```python
from build123d import *

# Parameters (mm, degrees)
SKETCH1_R           = 9
BOSS_EXTRUDE1_DEPTH = 14
SKETCH2_R           = 27.5
SKETCH2_R_2         = 15
BOSS_EXTRUDE2_DEPTH = 22.5
SKETCH3_R           = 27.5
SKETCH3_R_2         = 15
BOSS_EXTRUDE3_DEPTH = 22.5
BOSS_EXTRUDE4_DEPTH = 7.5
BOSS_EXTRUDE9_DEPTH = 7.5


with BuildPart() as part:
    # Sketch1 → Boss-Extrude1 (new body)
    with BuildSketch(Plane(origin=(0, 0, 0), x_dir=(1, 0, 0), z_dir=(0, 1, 0))):
        with BuildLine():
            Line((153.801246265, 0), (225.801246265, 0))
            ThreePointArc((225.801246265, 0), (232.872314076, 2.928932188), (235.801246265, 10))
            Line((235.801246265, 10), (235.801246265, 132))
            ThreePointArc((235.801246265, 132), (232.872314076, 139.071067812), (225.801246265, 142))
            Line((225.801246265, 142), (153.801246265, 142))
            ThreePointArc((153.801246265, 142), (146.730178453, 139.071067812), (143.801246265, 132))
            Line((143.801246265, 132), (143.801246265, 10))
            ThreePointArc((143.801246265, 10), (146.730178453, 2.928932188), (153.801246265, 0))
        make_face()
        with Locations(Location((164.801246265, 22.845020392, 0), (0, 0, 270))):
            Circle(SKETCH1_R, mode=Mode.SUBTRACT)
        with Locations(Location((214.801246265, 22.845020392, 0), (0, 0, 270))):
            Circle(SKETCH1_R, mode=Mode.SUBTRACT)
        with Locations(Location((214.801246265, 118.829727622, 0), (0, 0, 270))):
            Circle(SKETCH1_R, mode=Mode.SUBTRACT)
        with Locations(Location((164.801246265, 118.829727622, 0), (0, 0, 270))):
            Circle(SKETCH1_R, mode=Mode.SUBTRACT)
    extrude(amount=-BOSS_EXTRUDE1_DEPTH)



with BuildPart() as body_2:
    # Sketch2 → Boss-Extrude2 (new body)
    with BuildSketch(Plane.XY.offset(-71)):
        with Locations(Location((189.801246265, 58, 0), (0, 0, 180))):
            Circle(SKETCH2_R)
        with Locations(Location((189.801246265, 58, 0), (0, 0, 180))):
            Circle(SKETCH2_R_2, mode=Mode.SUBTRACT)
    extrude(amount=BOSS_EXTRUDE2_DEPTH)

    # Sketch3 → Boss-Extrude3 (add)
    with BuildSketch(Plane(origin=(0, 0, -71), x_dir=(-1, 0, 0), z_dir=(0, 0, -1))):
        with Locations((-189.801246265, 58)):
            Circle(SKETCH3_R)
        with Locations((-189.801246265, 58)):
            Circle(SKETCH3_R_2, mode=Mode.SUBTRACT)
    extrude(amount=BOSS_EXTRUDE3_DEPTH)


with BuildPart() as part_1:
    add(part.part)

    add(body_2.part)  # Boss-Extrude4 merges body 2
    # Sketch4 → Boss-Extrude4 (add, symmetric)
    with BuildSketch(Plane.XY.offset(-71)):
        with BuildLine():
            Line((143.801246265, 0), (235.801246265, 0))
            Line((235.801246265, 0), (235.801246265, 17.16449016))
            Line((235.801246265, 17.16449016), (217.301246265, 58))
            ThreePointArc((217.301246265, 58), (189.801246265, 30.5), (162.301246265, 58))
            Line((162.301246265, 58), (143.801246265, 17.16449016))
            Line((143.801246265, 17.16449016), (143.801246265, 0))
        make_face()
    extrude(amount=BOSS_EXTRUDE4_DEPTH, both=True)

    # Sketch6 → Boss-Extrude9 (add, symmetric)
    with BuildSketch(Plane.ZY.offset(-189.801246265)):
        Polygon((-119.5, 0), (-78.5, 0), (-76.506871872, 0), (-76.506871872, 30.5), (-76.506871872, 32.905088901), (-93.5, 32.905088901), align=None)
        Polygon((-22.5, 0), (-63.5, 0), (-65.39508201, 0), (-65.39508201, 32.905088901), (-48.424150578, 32.905088901), align=None)
    extrude(amount=BOSS_EXTRUDE9_DEPTH, both=True)


solid = part_1.part
```
Part model, mm, in its own coordinate system. A direction names the side the tool comes from. Coordinates: 2 decimals unless noted, no trailing zeros. Order: outer loops, then holes, each group sorted by start corner. A loop starts at its lowest first (then second) coordinate and runs counter-clockwise, first axis right, second up. Notation, with made-up numbers: (71, 38.5) - (107, 38.5) arc R9 cw to (107, 45.5) - close; hole circle Ø3 at (52.25, 70.5). An arc over 180 degrees is marked (long way). Return JSON: item names as keys, results as strings. Group by question number.
Item 1: Cut at C-C (y = 46.5). List the corners of the cut face in (x, z).
Item 2: Pin check, flat tips, straight feed: pin 1 (19 mm diameter, centred on x = 210, z = -21.5, fed in from +Y); pin 2 (1.5 mm diameter, centred on x = 176, z = -60.5, fed in from +Y); pin 3 (1 mm diameter, centred on x = 194.5, y = 37, fed in from +Z). Stop position of each tip, or through.
Item 3: Pull direction X, two halves, no side cores. Call faces 1 (the face through (204.787, 58.66, -70.685)), 2 (the face through (143.801, -5, -70)), 3 (the face through (232.95, -6.9, -138.99)): pulls with the +X half, pulls with the -X half, needs draft (parallel to the pull), parting line crosses it, or undercut.
Item 4: Cut at B-B (x = 194.5). List the corners of the cut face in (y, z), plus the area to 3 significant figures.
Item 5: Cut at A-A (z = -56). List the corners of the cut face in (x, y).
Item 6: Which spindle directions (+Z, -Z, +X, -X, +Y, -Y) get a long thin tool onto all of the face, cutting with end or side? Do faces 4 (the face through (197.301, 13, -47)), 5 (the face through (232.79, -6.9, -2.85)), 6 (the face through (216, 23, -78.5)). Say none if no direction does.
Item 7: Drill centre lines: probe 1 along X at (y, z) = (58, -70); probe 2 along X at (y, z) = (-1, -22); probe 3 along Y at (x, z) = (196.5, -14). Where is each one in solid material? Low to high. Write a range as from..to.
Item 8: Cut at D-D (z = -28). List the corners of the cut face in (x, y).
Check values:
{
 "1": {"outline": "(157.09, -78.5) - (164.82, -78.5) - (164.82, -93.5) - (180.17, -93.5) - (180.17, -48.5) - (164.82, -48.5) - (164.82, -63.5) - (157.09, -63.5) - close; (199.43, -93.5) - (214.78, -93.5) - (214.78, -78.5) - (222.51, -78.5) - (222.51, -63.5) - (214.78, -63.5) - (214.78, -48.5) - (199.43, -48.5) - close"},
 "2": {"pin 1": "stops at y = 0", "pin 2": "stops at y = 82.21", "pin 3": "stops at z = -48.5"},
 "3": {"face 1": "undercut", "face 2": "pulls with the -X half", "face 3": "pulls with the +X half"},
 "4": {"outline": "(-14, -142) - (0, -142) - (0, -119.5) - (32.91, -93.5) - (43.75, -93.5) - (43.75, -48.5) - (32.91, -48.5) - (32.91, -48.42) - (0, -22.5) - (0, 0) - (-14, 0) - close; (72.25, -93.5) - (85.1, -93.5) - (85.1, -48.5) - (72.25, -48.5) - close", "area": "5,390 mm2"},
 "5": {"outline": "(143.8, -14) - (235.8, -14) - (235.8, 0) - (197.3, 0) - (197.3, 31.54) arc R27.5 ccw (long way) to (182.3, 31.54) - (182.3, 0) - (143.8, 0) - close; hole circle Ø30 at (189.8, 58)"},
 "6": {"face 4": "+Z, +X", "face 5": "+Z, +X, +Y, -Y", "face 6": "-Z, +X"},
 "7": {"probe 1": "x = 162.3..174.8, 204.8..217.3", "probe 2": "x = 143.8..155.84, 173.76..205.84, 223.76..235.8", "probe 3": "y = -14..0"},
 "8": {"outline": "(143.8, -14) - (157.42, -14) - (157.42, 0) - (143.8, 0) - close; (172.18, -14) - (207.42, -14) - (207.42, 0) - (197.3, 0) - (197.3, 6.98) - (182.3, 6.98) - (182.3, 0) - (172.18, 0) - close; (222.18, -14) - (235.8, -14) - (235.8, 0) - (222.18, 0) - close"}
}
